from build123d import *

# Parameters (mm, degrees)
BASE_EXTRU_MINCE_DEPTH = 400
CONG_1_R               = 1.5
CONG_2_R               = 0.5


with BuildPart() as part:
    # Esquisse1 → Base-Extru.-Mince (new body)
    with BuildSketch(Plane.XY):
        Polygon((-6.25, 10), (-9.75, 10), (-9.75, 0.5), (-5, 0.5), (-5, 0), (5, 0), (5, 0.5), (9.75, 0.5), (9.75, 10), (6.25, 10), (6.25, 9), (8.75, 9), (8.75, 1.5), (4, 1.5), (4, 1), (-4, 1), (-4, 1.5), (-8.75, 1.5), (-8.75, 9), (-6.25, 9), align=None)
    extrude(amount=BASE_EXTRU_MINCE_DEPTH)

    # Congé1
    cong_1_edges = [part.edges().sort_by_distance(p)[0] for p in [
        (-9.75, 10, 200),
        (-9.75, 0.5, 200),
        (9.75, 0.5, 200),
        (9.75, 10, 200),
    ]]
    fillet(cong_1_edges, radius=CONG_1_R)

    # Congé2
    cong_2_edges = [part.edges().sort_by_distance(p)[0] for p in [
        (-8.75, 9, 200),
        (-8.75, 1.5, 200),
        (8.75, 1.5, 200),
        (8.75, 9, 200),
    ]]
    fillet(cong_2_edges, radius=CONG_2_R)


solid = part.part
Here's how the part is built. I have some questions about the finished solid (model axes, mm). A direction names the side the tool comes from. Coordinates: 2 decimals unless noted, no trailing zeros. Order: outer loops, then holes, each group sorted by start corner. A loop starts at its lowest first (then second) coordinate and runs counter-clockwise, first axis right, second up.
Item 1: I need wall thicknesses on line 1 (X direction, y = 8, z = 72.5); line 2 (X direction, y = 1.75, z = 264); line 3 (Y direction, x = -7.5, z = 211). Which ranges of each line are inside material? Lowest first, please.
Result sheet:
line 1: x = -9.75 to -8.75, 8.75 to 9.75
line 2: x = -9.73 to -8.68, 8.68 to 9.73
line 3: y = 0.5 to 1.5, 9 to 10
Item 2: For P1, Ø3, axis at x = 7, y = 4.5, coming from the -Z side; P2, Ø0.6, axis at x = -7.5, z = 206.5, coming from the -Y side; P3, Ø0.6, axis at y = 1.5, z = 100.5, coming from the -X side; P4, Ø9, axis at x = 0.5, z = 232, coming from the +Y side, each with a flat end and sliding along its axis, tell me the tip position at first contact or that it passes through.
Result sheet:
P1: passes through
P2: stops at y = 0.5
P3: stops at x = -9.74
P4: stops at y = 1.5
Item 3: If we mould it in two halves opening along X, with no side actions, what happens to faces 3 (the face through (0, 0.6, 400)), 4 (the face through (-9.75, 5, 197)), 5 (the face through (0, 1, 197)), 6 (the face through (-8.75, 5, 197))? For each: +X half, -X half, draft (parallel to the pull), parting line (faces both ways), or undercut.
Result sheet:
face 3: draft
face 4: -X half
face 5: undercut
face 6: undercut
Item 4: If we section it at B-B on y = 3.75: List the corners of the cut face in (x, z) for me.
Result sheet:
outline: (-9.75, 0) - (-8.75, 0) - (-8.75, 400) - (-9.75, 400) - close; (8.75, 0) - (9.75, 0) - (9.75, 400) - (8.75, 400) - close
Item 5: If we section it at A-A on z = 351: List the corners of the cut face in (x, y) for me.
Result sheet:
outline: (-9.75, 2) arc R1.5 ccw to (-8.25, 0.5) - (-5, 0.5) - (-5, 0) - (5, 0) - (5, 0.5) - (8.25, 0.5) arc R1.5 ccw to (9.75, 2) - (9.75, 8.5) arc R1.5 ccw to (8.25, 10) - (6.25, 10) - (6.25, 9) - (8.25, 9) arc R0.5 cw to (8.75, 8.5) - (8.75, 2) arc R0.5 cw to (8.25, 1.5) - (4, 1.5) - (4, 1) - (-4, 1) - (-4, 1.5) - (-8.25, 1.5) arc R0.5 cw to (-8.75, 2) - (-8.75, 8.5) arc R0.5 cw to (-8.25, 9) - (-6.25, 9) - (-6.25, 10) - (-8.25, 10) arc R1.5 ccw to (-9.75, 8.5) - close
Item 6: For faces 1 (the face through (8.75, 5, 197)), 2 (the face through (0, 0, 197)), which set-ups out of +Z, -Z, +X, -X, +Y, -Y let a thin tool reach every point of the face, with its end or its side?
Result sheet:
face 1: +Z, -Z
face 2: +Z, -Z, +X, -X, -Y
Item 7: If we section it at C-C on x = 0: List the corners of the cut face in (y, z) for me.
Result sheet:
outline: (0, 0) - (1, 0) - (1, 400) - (0, 400) - close
